Could you check a few things on this model? Use its own coordinates, in mm. Face numbers are marked on the shaded views. A direction names the side the tool comes from. Coordinates: 2 decimals unless noted, no trailing zeros. Order: outer loops, then holes, each group sorted by start corner. A loop starts at its lowest first (then second) coordinate and runs counter-clockwise, first axis right, second up. Notation, with made-up numbers: (19, -26.75) - (34, -26.75) arc R36 cw to (34, 10.25) - close; hole circle Ø3 at (-23.75, 41). An arc over 180 degrees is marked (long way). One line per item, written item: value.
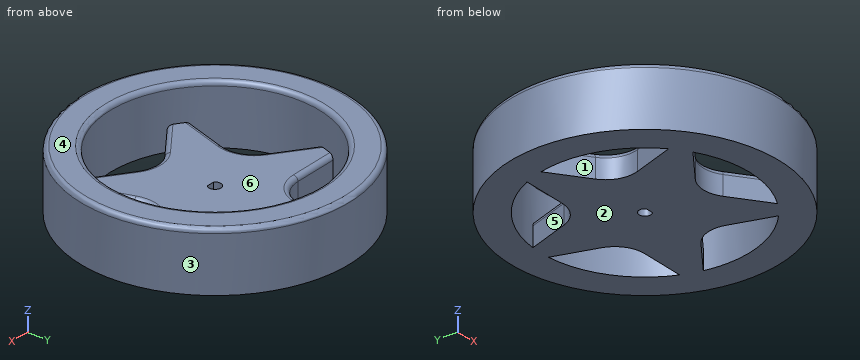
Autodesk Fusion 360 part; units mm, degrees
sketch "Esboço1" plane through (0, 0, 0) normal (0, 0, 1) x (1, 0, 0)
  circle A0 centre (0, 0) radius 45
  circle A1 centre (0, 0) radius 2
  circle A2 centre (0, 0) radius 35
  line L0 (-7.858, 20.8156) -> (0, 45)
  line L1 (-42.7975, 13.9058) -> (-17.3686, 13.9058)
  arc A3 (-17.3686, 13.9058) -> (-7.858, 20.8156) centre (-17.3686, 23.9058) ccw
  line L2 (0, 45) -> (7.858, 20.8156)
  line L3 (42.7975, 13.9058) -> (17.3686, 13.9058)
  arc A4 (7.858, 20.8156) -> (17.3686, 13.9058) centre (17.3686, 23.9058) ccw
  line L4 (-42.7975, 13.9058) -> (-22.2251, -1.041)
  line L5 (-26.4503, -36.4058) -> (-18.5923, -12.2214)
  arc A5 (-18.5923, -12.2214) -> (-22.2251, -1.041) centre (-28.1029, -9.1312) ccw
  line L6 (22.2251, -1.041) -> (42.7975, 13.9058)
  line L7 (26.4503, -36.4058) -> (18.5923, -12.2214)
  arc A6 (22.2251, -1.041) -> (18.5923, -12.2214) centre (28.1029, -9.1312) ccw
  line L8 (5.8779, -21.459) -> (26.4503, -36.4058)
  line L9 (-26.4503, -36.4058) -> (-5.8779, -21.459)
  arc A7 (5.8779, -21.459) -> (-5.8779, -21.459) centre (0, -29.5492) ccw
  line L10 (0, -1.5) -> (-1.3229, -1.5)
  line L11 (0, -1.5) -> (1.3229, -1.5)
  dimension "d1" = 10
  dimension "d2" = 10
  dimension "d3" = 10
  dimension "d4" = 10
  dimension "d5" = 10
extrude "Extrusão1" add sketch "Esboço1" along normal blind 20 contours A0 A2 L6 L7 | A0 A2 L2 L3 | A2 L3 L6 | A2 L7 L8 | A0 A2 L8 L9 | A0 A2 L0 L1 | A2 L0 L2 | A0 A2 L4 L5 | A2 L5 L9 | A2 L1 L4
extrude "Extrusão2" add sketch "Esboço1" along normal blind 8 contours A2 L0 L1 A3 L2 L3 A4 L4 L5 A5 L6 L7 A6 L8 L9 A7 | A1 L10 L11 picked at (-0.096, -1.8264)
fillet "Arredondamento1" radius 1.5 17 edges at (-41.9547, -16.2727, 20) (-32.6315, 12.6565, 20) (-28.1917, 3.294, 8) (-18.5923, -6.041, 8) (-20.8714, -19.2356, 8) (-5.5789, 27.8298, 8) (-11.4907, 15.8156, 8) (-24.7438, 13.9058, 8) (24.7438, 13.9058, 8) (11.4907, 15.8156, 8) (5.5789, 27.8298, 8) (20.8714, -19.2356, 8) (18.5923, -6.041, 8) (28.1917, 3.294, 8) (-11.8445, -25.794, 8) (0, -19.5492, 8) (11.8445, -25.794, 8)
sketch "Esboço2" plane through (0, 0, 20) normal (0, 0, 1) x (-1, 0, 0)
  circle A0 centre (0, 0) radius 43.5
  circle A1 centre (0, 0) radius 36.5
Item 1: I want a section at B-B on z = 11.5. Please give me the cut outline in (x, y).
Conclusion:
outline: circle Ø90 at (0, 0); hole circle Ø70 at (0, 0)
Item 2: I want a section at A-A on x = 0. Please give me the cut outline in (y, z), then the cut area to 3 significant figures.
Conclusion:
outline: (-45, 0) - (-35, 0) - (-35, 18.5) arc R1.5 ccw to (-36.5, 20) - (-43.5, 20) arc R1.5 ccw to (-45, 18.5) - close; (-19.55, 0) - (-1.5, 0) - (-1.5, 8) - (-18.05, 8) arc R1.5 ccw to (-19.55, 6.5) - close; (2, 0) - (45, 0) - (45, 18.5) arc R1.5 ccw to (43.5, 20) - (36.5, 20) arc R1.5 ccw to (35, 18.5) - (35, 8) - (2, 8) - close
area: 806 mm²
Item 3: If I drill on probe 1 along Y at (x, z) = (0, 4); probe 2 along X at (y, z) = (0, 8.5); probe 3 along X at (y, z) = (-1, 3.25), over which ranges is the centre line in solid material (lowest first)?
Conclusion:
probe 1: -45 to -35, -19.55 to -1.5, 2 to 45
probe 2: -45 to -35, 35 to 45
probe 3: -44.99 to -34.99, -22.28 to -1.73, 1.73 to 22.28, 34.99 to 44.99
Item 4: I'm going to push flat-ended pins straight in: pin 1 Ø5 at (x, z) = (-16.5, 16) entering from -Y; pin 2 Ø1.5 at (y, z) = (-21.5, 9) entering from -X; pin 3 Ø4 at (x, z) = (23.5, 9.5) entering from -Y. Where does each tip first touch, or does it pass through?
Conclusion:
pin 1: y = -42.77
pin 2: x = -39.93
pin 3: y = -39.53
Item 5: Thinking about a two-plate mould opening in Y: for the marked faces 1, 2 and 3, which applies, pulls with the +Y half, pulls with the -Y half, needs draft (parallel to the pull), parting line crosses it, or undercut?
Conclusion:
face 1: undercut
face 2: needs draft
face 3: parting line crosses it
Item 6: I want a section at C-C on y = -7.5. Give the number of separate pieces and of enclosed holes in the cut face, then the cut area to 3 significant figures.
Conclusion:
separate pieces: 3
enclosed holes: 0
area: 696 mm²
Item 7: For the marked faces 4, 5 and 6, which set-ups out of +Z, -Z, +X, -X, +Y, -Y let a thin tool reach every point of the face, with its end or its side?
Conclusion:
face 4: +Z, +X, -X, +Y, -Y
face 5: +Z, -Z
face 6: +Z
